from build123d import *

# Parameters (mm, degrees)
SKETCH_1_W           = 200
SKETCH_1_H           = 200
EXTRUDE_1_DEPTH      = 191
SHELL_1_T            = -20
SKETCH_4_5_R         = 51
CUT_EXTRUDE_6_DEPTH  = 191
SKETCH_4_R           = 8.642247924
CUT_EXTRUDE_7_DEPTH  = 50
SKETCH_4_10_R        = 57.15
CUT_EXTRUDE_9_DEPTH  = 50
CUT_EXTRUDE_START    = -171
SKETCH_4_11_R        = 4
CUT_EXTRUDE_10_DEPTH = 50
SKETCH_9_W           = 200
SKETCH_9_H           = 200
EXTRUDE_3_DEPTH      = 32
SKETCH_10_R          = 72.5
CUT_EXTRUDE_11_DEPTH = 2
SKETCH_11_R          = 72
CUT_EXTRUDE_13_DEPTH = 30
SKETCH_11_3_W        = 200
SKETCH_11_3_H        = 200
SKETCH_11_3_R        = 77
CUT_EXTRUDE_14_DEPTH = 5
SKETCH_14_W          = 25
SKETCH_14_H          = 200
EXTRUDE_4_DEPTH      = 25
SKETCH_15_R          = 5.5
CUT_EXTRUDE_15_DEPTH = 25
SKETCH_16_R          = 3
CUT_EXTRUDE_16_DEPTH = 20
FILLET_1_R           = 0.5


with BuildPart() as part:
    # 草图1 → 凸台-拉伸1 (new body)
    with BuildSketch(Plane.XY):
        with Locations((43.238558972, -58.914961101)):
            Rectangle(SKETCH_1_W, SKETCH_1_H)
    extrude(amount=EXTRUDE_1_DEPTH)

    # 抽壳1
    shell_1_openings = [part.faces().sort_by_distance(p)[0] for p in [
        (43.238558972, -158.914961101, 95.5),
    ]]
    offset(amount=SHELL_1_T, openings=shell_1_openings, kind=Kind.INTERSECTION)

    # 草图4<5> → 切除-拉伸6 (cut)
    with BuildSketch(Plane.XY.offset(191)):
        with Locations((43.238558972, -58.914961101)):
            Circle(SKETCH_4_5_R)
    extrude(amount=-CUT_EXTRUDE_6_DEPTH, mode=Mode.SUBTRACT)

    # 草图4 → 切除-拉伸7 (cut)
    with BuildSketch(Plane.XY.offset(191)):
        with Locations((-27.472119147, 11.795717018)):
            Circle(SKETCH_4_R)
        with Locations((113.949237091, 11.795717018)):
            Circle(SKETCH_4_R)
        with Locations((113.949237091, -129.625639219)):
            Circle(SKETCH_4_R)
        with Locations((-27.472119147, -129.625639219)):
            Circle(SKETCH_4_R)
    extrude(amount=-CUT_EXTRUDE_7_DEPTH, mode=Mode.SUBTRACT)

    # 草图4<10> → 切除-拉伸9 (cut)
    with BuildSketch(Plane.XY.offset(191)):
        with Locations((43.238558972, -58.914961101)):
            Circle(SKETCH_4_10_R)
    extrude(amount=-CUT_EXTRUDE_9_DEPTH, mode=Mode.SUBTRACT)

    # 草图4<11> → 切除-拉伸10 (cut)
    with BuildSketch(Plane.XY.offset(191).offset(CUT_EXTRUDE_START)):
        with Locations(Location((-17.761441028, -58.914961101, 0), (0, 0, 180))):
            Circle(SKETCH_4_11_R)
        with Locations(Location((12.738558972, -6.08741147, 0), (0, 0, 180))):
            Circle(SKETCH_4_11_R)
        with Locations(Location((73.738558972, -6.08741147, 0), (0, 0, 180))):
            Circle(SKETCH_4_11_R)
        with Locations(Location((104.238558972, -58.914961101, 0), (0, 0, 180))):
            Circle(SKETCH_4_11_R)
        with Locations(Location((73.738558972, -111.742510731, 0), (0, 0, 180))):
            Circle(SKETCH_4_11_R)
        with Locations(Location((12.738558972, -111.742510731, 0), (0, 0, 180))):
            Circle(SKETCH_4_11_R)
    extrude(amount=-CUT_EXTRUDE_10_DEPTH, mode=Mode.SUBTRACT)

    # 草图9 → 凸台-拉伸3 (add)
    with BuildSketch(Plane(origin=(0, 0, 0), x_dir=(-1, 0, 0), z_dir=(0, 0, -1))):
        with Locations((-43.238558972, -58.914961101)):
            Rectangle(SKETCH_9_W, SKETCH_9_H)
    extrude(amount=EXTRUDE_3_DEPTH)

    # 草图10 → 切除-拉伸11 (cut)
    with BuildSketch(Plane.XY):
        with Locations((43.238558972, -57.634762562)):
            Circle(SKETCH_10_R)
    extrude(amount=-CUT_EXTRUDE_11_DEPTH, mode=Mode.SUBTRACT)

    # 草图11 → 切除-拉伸13 (cut)
    with BuildSketch(Plane(origin=(0, 0, -32), x_dir=(-1, 0, 0), z_dir=(0, 0, -1))):
        with Locations((-43.238558972, -58.914961101)):
            Circle(SKETCH_11_R)
    extrude(amount=-CUT_EXTRUDE_13_DEPTH, mode=Mode.SUBTRACT)

    # 草图11<3> → 切除-拉伸14 (cut)
    with BuildSketch(Plane(origin=(0, 0, -32), x_dir=(-1, 0, 0), z_dir=(0, 0, -1))):
        with Locations((-43.238558972, -58.914961101)):
            Rectangle(SKETCH_11_3_W, SKETCH_11_3_H)
        with Locations((-43.238558972, -58.914961101)):
            Circle(SKETCH_11_3_R, mode=Mode.SUBTRACT)
    extrude(amount=-CUT_EXTRUDE_14_DEPTH, mode=Mode.SUBTRACT)

    # 草图14 → 凸台-拉伸4 (add)
    with BuildSketch(Plane(origin=(0, 0, -27), x_dir=(-1, 0, 0), z_dir=(0, 0, -1))):
        with Locations((-155.738558972, -58.914961101)):
            Rectangle(SKETCH_14_W, SKETCH_14_H)
        with Locations((69.261441028, -58.914961101)):
            Rectangle(SKETCH_14_W, SKETCH_14_H)
    extrude(amount=-EXTRUDE_4_DEPTH)

    # 草图15 → 切除-拉伸15 (cut)
    with BuildSketch(Plane.XY.offset(-2)):
        with Locations((-71.761441028, 21.085038899)):
            Circle(SKETCH_15_R)
        with Locations(Location((-71.761441028, -138.914961101, 0), (0, 0, 180))):
            Circle(SKETCH_15_R)
        with Locations((158.238558972, 21.085038899)):
            Circle(SKETCH_15_R)
        with Locations((158.238558972, -138.914961101)):
            Circle(SKETCH_15_R)
    extrude(amount=-CUT_EXTRUDE_15_DEPTH, mode=Mode.SUBTRACT)

    # 草图16 → 切除-拉伸16 (cut)
    with BuildSketch(Plane.XZ.offset(158.914961101)):
        with Locations((133.238558972, 181)):
            Circle(SKETCH_16_R)
        with Locations(Location((-46.761441028, 181, 0), (0, 0, 180))):
            Circle(SKETCH_16_R)
        with Locations((-46.761441028, -17)):
            Circle(SKETCH_16_R)
        with Locations((133.238558972, -17)):
            Circle(SKETCH_16_R)
    extrude(amount=-CUT_EXTRUDE_16_DEPTH, mode=Mode.SUBTRACT)

    # 圆角1
    fillet_1_edges = [part.edges().sort_by_distance(p)[0] for p in [
        (115.238558972, -58.914961101, -32),
        (120.238558972, -58.914961101, -32),
        (-13.911441028, -58.914961101, 191),
    ]]
    fillet(fillet_1_edges, radius=FILLET_1_R)


solid = part.part
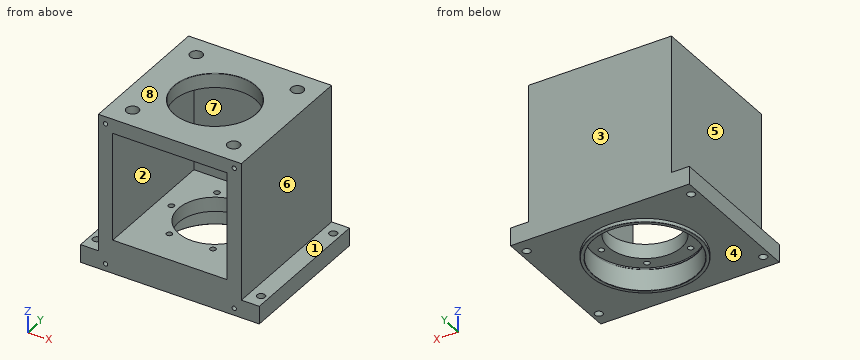
Geometry: final body of the model. Coordinates: model frame, mm. Face numbers are marked on the shaded views. A direction names the side the tool comes from. Give positions to 0.01 mm unless a question says otherwise; leave off trailing zeros. Loops run counter-clockwise (first coordinate to the right, second up) from the corner with the lowest first, then second, coordinate; pieces in that order, holes last. Notation, with made-up numbers: (22, -2.5) - (61, -2.5) arc R29 ccw to (61, 27.5) - close; hole circle Ø8 at (9.25, 33). An arc over 180 degrees is marked (long way). Answer as CSV lines item,"result". Start each with the question number.
1. Section A-A, the plane z = 37. Return loops of the section in (x, y), plus the area to 3 significant figures.
2. Section B-B, the plane x = 41. Give the number of separate pieces and of enclosed holes in the cut face, plus the area to 3 significant figures.
3. Pin query (flat end, axial travel): P1, Ø6, axis at x = -2.5, z = 83.5, coming from the -Y side; P2, Ø9, axis at x = -71.76, y = -138.91, coming from the +Z side; P3, Ø1.5, axis at y = -89, z = 89.5, coming from the +X side; P4, Ø12, axis at x = 137.5, y = -42.5, coming from the -Z side. Return the tip coordinate at first contact, or that it passes through.
4. Ray query, L1, parallel to X at y = -71, z = 150; L2, parallel to Y at x = 9.5, z = 2.5; L3, parallel to Z at x = 85, y = -133. Return the intervals inside material, ascending.
5. Reachability of the marked faces 4, 5, 6, 7 and 8 from +Z, -Z, +X, -X, +Y, -Y: full face, straight path, thin tool, end or side. Return the list, or none.
6. Draft query along Z for the marked faces 1, 2 and 3. Return one class per face: released by +Z, released by -Z, zero draft, split by the parting line, or undercut.
Answers:
1,outline,"(-56.76, -158.91) - (-36.76, -158.91) - (-36.76, 21.09) - (123.24, 21.09) - (123.24, -158.91) - (143.24, -158.91) - (143.24, 41.09) - (-56.76, 41.09) - close"
1,area,"11,200 mm2"
2,separate pieces,"3"
2,enclosed holes,"0"
2,area,"8,260 mm2"
3,P1,"stops at y = 21.09"
3,P2,"passes through"
3,P3,"stops at x = 143.24"
3,P4,"stops at z = -27"
4,L1,"x = -56.76 to -36.76, 123.24 to 143.24"
4,L2,"y = -158.91 to -114.09, -109.39 to -97.16, -20.67 to -8.44, -3.74 to 41.09"
4,L3,"z = -27 to 20, 171 to 191"
5,face 4,"-Z"
5,face 5,"+Z, -X, +Y, -Y"
5,face 6,"+Z, +X, +Y, -Y"
5,face 7,"-Y"
5,face 8,"+Z, +X, -X, +Y, -Y"
6,face 1,"released by +Z"
6,face 2,"undercut"
6,face 3,"zero draft"
